Answer from the drawing. Dimensions are ordinates in mm from the lowest x, y and z of the part. Round coordinates to 2 decimals unless told otherwise and drop trailing zeros. Loops run counter-clockwise (first coordinate to the right, second up) from the corner with the lowest first, then second, coordinate; pieces in that order, holes last.
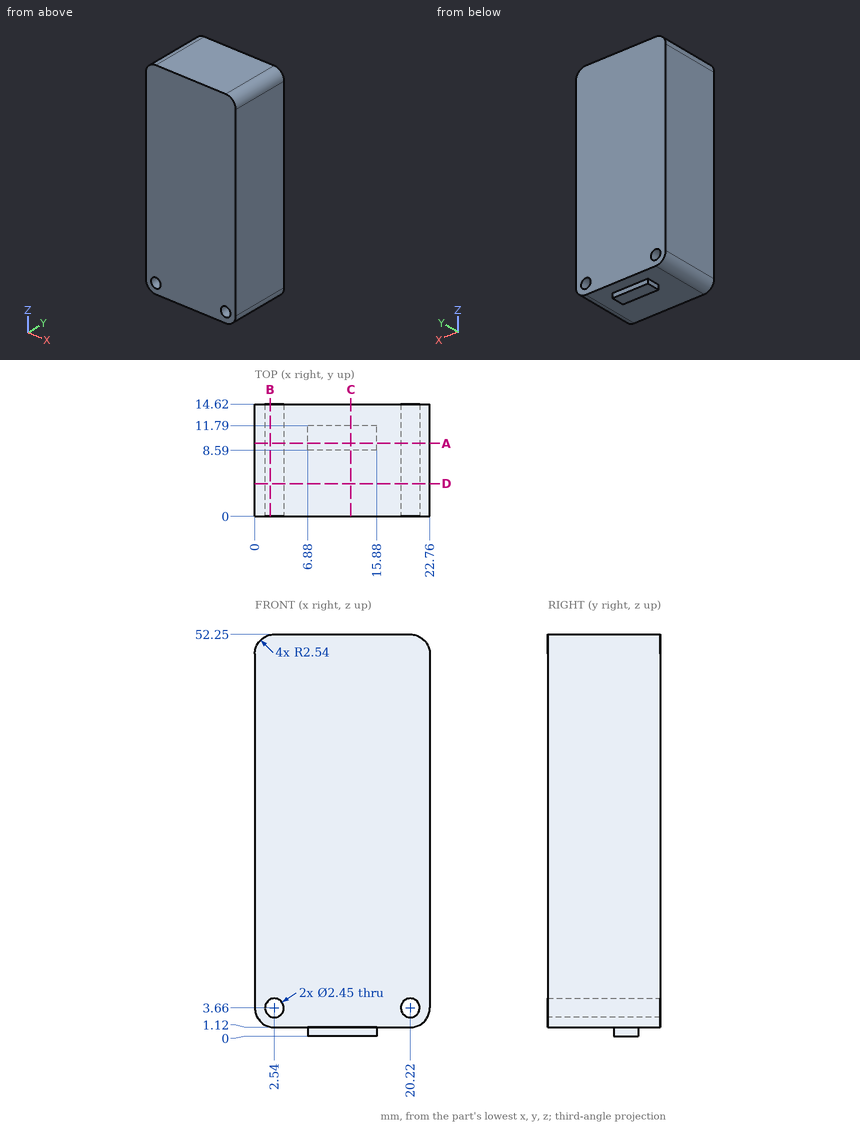
Item 1: Section D-D, the plane y = 4.25 is taken. Give the vertices of the cut face in (x, z) (3 decimals).
Item 2: Section B-B, the plane x = 2 is taken. Give the vertices of the cut face in (y, z), plus the area to 3 significant figures.
Item 3: Each of these flat-tipped pins is pushed along its axis until it touches: P1, Ø0.6, axis at x = 10.5, z = 0.5, coming from the +Y side; P2, Ø1.5, axis at x = 5, z = 7.5, coming from the -Y side; P3, Ø5, axis at x = 11.5, y = 1.5, coming from the -Z side; P4, Ø1.2, axis at y = 10, z = 1, coming from the -X side. Where does it stop, or does it pass through?
Item 4: Section A-A, the plane y = 9.5 is taken. Give the vertices of the cut face in (x, z) (3 decimals).
Item 5: Section C-C, the plane x = 12.5 is taken. Give the vertices of the cut face in (y, z).
Item 6: Straight lines are drawn through the part: line 1 (X direction, y = 6.75, z = 3.66) (3 decimals); line 2 (Z direction, x = 2.54, y = 8.75) (3 decimals); line 3 (X direction, y = 5.5, z = 4). For each, find the intervals that lie inside material, in ascending order.
Answer below:
1. outline: (0, 3.66) arc R2.54 ccw to (2.54, 1.12) - (20.22, 1.12) arc R2.54 ccw to (22.76, 3.66) - (22.76, 49.71) arc R2.54 ccw to (20.22, 52.25) - (2.54, 52.25) arc R2.54 ccw to (0, 49.71) - close; hole circle Ø2.45 at (2.54, 3.66); hole circle Ø2.45 at (20.22, 3.66)
2. outline: (0, 1.18) - (14.62, 1.18) - (14.62, 2.56) - (0, 2.56) - close; (0, 4.76) - (14.62, 4.76) - (14.62, 52.19) - (0, 52.19) - close
2. area: 714 mm2
3. P1: stops at y = 11.79
3. P2: stops at y = 0
3. P3: stops at z = 1.12
3. P4: stops at x = 1.05
4. outline: (0, 3.66) arc R2.54 ccw to (2.54, 1.12) - (6.88, 1.12) - (6.88, 0) - (15.88, 0) - (15.88, 1.12) - (20.22, 1.12) arc R2.54 ccw to (22.76, 3.66) - (22.76, 49.71) arc R2.54 ccw to (20.22, 52.25) - (2.54, 52.25) arc R2.54 ccw to (0, 49.71) - close; hole circle Ø2.45 at (2.54, 3.66); hole circle Ø2.45 at (20.22, 3.66)
5. outline: (0, 1.12) - (8.59, 1.12) - (8.59, 0) - (11.79, 0) - (11.79, 1.12) - (14.62, 1.12) - (14.62, 52.25) - (0, 52.25) - close
6. line 1: x = 0 to 1.315, 3.765 to 18.995, 21.445 to 22.76
6. line 2: z = 1.12 to 2.435, 4.885 to 52.25
6. line 3: x = 0 to 1.36, 3.72 to 19.04, 21.4 to 22.76
